from build123d import *

# Parameters (mm, degrees)
BOSS_EXTRUDE1_DEPTH = 114.3
BOSS_EXTRUDE2_DEPTH = 19.05


with BuildPart() as part:
    # Sketch2 → Boss-Extrude1 (new body)
    with BuildSketch(Plane.XY):
        with BuildLine():
            Line((-7.31960848, -7.119729616), (7.399296286, -7.119729616))
            ThreePointArc((7.399296286, -7.119729616), (10.453843903, 0.248435463), (7.399296286, 7.616600541))
            Line((7.399296286, 7.616600541), (-7.31960848, 7.616600541))
            ThreePointArc((-7.31960848, 7.616600541), (-10.374156097, 0.248435463), (-7.31960848, -7.119729616))
        make_face()
    extrude(amount=-BOSS_EXTRUDE1_DEPTH)

    # Sketch1 → Boss-Extrude2 (add)
    with BuildSketch(Plane.XY):
        with BuildLine():
            Line((-21.701618149, -25.338055696), (21.501073099, -25.338055696))
            ThreePointArc((21.501073099, -25.338055696), (24.195149936, -24.222132532), (25.311073099, -21.528055696))
            Line((25.311073099, -21.528055696), (25.311073099, 21.674635553))
            ThreePointArc((25.311073099, 21.674635553), (24.195149936, 24.368712389), (21.501073099, 25.484635553))
            Line((21.501073099, 25.484635553), (-21.701618149, 25.484635553))
            ThreePointArc((-21.701618149, 25.484635553), (-24.395694985, 24.368712389), (-25.511618149, 21.674635553))
            Line((-25.511618149, 21.674635553), (-25.511618149, -21.528055696))
            ThreePointArc((-25.511618149, -21.528055696), (-24.395694985, -24.222132532), (-21.701618149, -25.338055696))
        make_face()
    extrude(amount=-BOSS_EXTRUDE2_DEPTH)


solid = part.part
Source: CAD feature listing. Evaluate the final solid. Frame: model axes, mm. A direction names the side the tool comes from. Coordinates: 2 decimals unless noted, no trailing zeros. Loops run counter-clockwise (first coordinate to the right, second up) from the corner with the lowest first, then second, coordinate; pieces in that order, holes last. Notation, with made-up numbers: (-29, 71.25) - (18, 71.25) arc R15 cw to (18, 99.25) - close; hole circle Ø6 at (63.5, 46.5). An arc over 180 degrees is marked (long way). One line per question, with ' | ' between items.
1) Section D-D, the plane x = 20. Return loops of the section in (y, z).
Report:
outline: (-25.34, -19.05) - (25.48, -19.05) - (25.48, 0) - (-25.34, 0) - close
2) Section A-A, the plane x = -5. Return loops of the section in (y, z), then the cut area to 3 significant figures.
Report:
outline: (-25.34, -19.05) - (-7.12, -19.05) - (-7.12, -114.3) - (7.62, -114.3) - (7.62, -19.05) - (25.48, -19.05) - (25.48, 0) - (-25.34, 0) - close | area: 2,370 mm²
3) Line query: line 1 along Z through (x, y) = (-2.5, 23); line 2 along Y through (x, z) = (0, -52.5); line 3 along X through (y, z) = (-5, -20.5). Output: solid intervals per line, ascending.
Report:
line 1: z = -19.05 to 0 | line 2: y = -7.12 to 7.62 | line 3: x = -8.95 to 9.03
4) Set-up query: faces 1 (the face through (0, -7.12, -66)), 2 (the face through (0, 7.617, -66)), 3 (the face through (-10.374, 0.363, -66.008)), 4 (the face through (10.453, 0.134, -66.008)). Return all of +Z, -Z, +X, -X, +Y, -Y with unobstructed straight access to the full face (end or side cutting, diameter ignored); none if empty.
Report:
face 1: -Z, +X, -X, -Y | face 2: -Z, +X, -X, +Y | face 3: -Z, -X | face 4: -Z, +X
5) First-contact query: P1, Ø10, axis at x = -17.5, z = -58, coming from the +Y side; P2, Ø16, axis at x = 0.5, z = -89, coming from the +Y side; P3, Ø2, axis at x = 8, y = -17, coming from the -Z side; P4, Ø2, axis at x = 1.5, y = -14, coming from the +Z side. Flat tips, straight axial feed; report the tip coordinate or a pass-through.
Report:
P1: passes through | P2: stops at y = 7.62 | P3: stops at z = -19.05 | P4: stops at z = 0
6) Section B-B, the plane y = -0.5. Return loops of the section in (x, z).
Report:
outline: (-25.51, -19.05) - (-10.35, -19.05) - (-10.35, -114.3) - (10.43, -114.3) - (10.43, -19.05) - (25.31, -19.05) - (25.31, 0) - (-25.51, 0) - close
7) Section C-C, the plane z = -102. Return loops of the section in (x, y), then the cut area to 3 significant figures.
Report:
outline: (-7.32, -7.12) - (7.4, -7.12) arc R10.41 ccw to (7.4, 7.62) - (-7.32, 7.62) arc R10.41 ccw to start | area: 279 mm²
